Autodesk Inventor part; units mm, degrees
ref_plane "Work Plane1" through (0, 4, 5) normal (0, 0, -1) x (-1, 0, 0)
ref_plane "YZ Plane" through (0, 0, 0) normal (1, 0, 0) x (0, 1, 0)
ref_plane "XZ Plane" through (0, 0, 0) normal (0, 1, 0) x (-1, 0, 0)
sketch "Sketch1" plane through (0, 0, 0) normal (0, 1, 0) x (-1, 0, 0)
  circle A0 centre (0, 0) radius 12.7
  dimension "d0" = 25.4
extrude "Extrusion1" add sketch "Sketch1" along normal blind 4
sketch "Sketch2" plane through (0, 4, 0) normal (0, 1, 0) x (1, 0, 0)
  circle A0 centre (0, 8.382) radius 1.524
  circle A1 centre (0, 0) radius 12.7
  circle A2 centre (-8.382, 0) radius 1.524
  circle A3 centre (0, -8.382) radius 1.524
  circle A4 centre (8.382, 0) radius 1.524
  dimension "d7" = 360
extrude "Extrusion2" cut sketch "Sketch2" along normal mid plane 8 contours A0 | A2 | A3 | A4
sketch "Sketch10" plane through (0, 0, 0) normal (0, -1, 0) x (1, 0, 0)
  circle A0 centre (0, 0) radius 12.7
  circle A1 centre (0, 0) radius 3.5
  dimension "d49" = 7
extrude "Extrusion9" cut sketch "Sketch10" against normal blind 2 contours A1
sketch "Sketch11" plane through (0, 4, 0) normal (0, 1, 0) x (1, 0, 0)
  circle A0 centre (0, 0) radius 3.5
  circle A1 centre (0, 0) radius 5
  circle A2 centre (0, 0) radius 2.625
  dimension "d52" = 10
  dimension "d53" = 5.25
extrude "Extrusion10" add sketch "Sketch11" along normal blind 6 contours A0 | A1
sketch "Sketch12" plane through (0, 10, 0) normal (0, 1, 0) x (1, 0, 0)
  line L0 (0, -1.3125) -> (-2.2733, -1.3125)
  circle A0 centre (0, 0) radius 2.625
  arc A1 (-2.2733, -1.3125) -> (2.2733, -1.3125) centre (0, 0) ccw
  line L1 (0, -1.3125) -> (2.2733, -1.3125)
  dimension "d56" = 1.3125
extrude "Extrusion11" add sketch "Sketch12" against normal up to surface (6 mm away) contours L1 A0 L0 picked at (1.3942, -1.4755)
ref_plane "Work Plane1" through (0, 4, 5) normal (0, 0, -1) x (-1, 0, 0)
sketch "Sketch13" plane through (0, 4, 5) normal (0, 0, -1) x (-1, 0, 0)
  line L0 (5, 6) -> (-5, 6)
  circle A0 centre (0, 3) radius 1.25
  point P0 (0, -4)
  dimension "d60" = 2.5
extrude "Extrusion12" cut sketch "Sketch13" along normal up to surface (3.6875 mm away)
properties part number "Horn_Attachment"
Check sheet for the modelled part. Datum: model origin and axes. Units: mm. A direction names the side the tool comes from. Round coordinates to 2 decimals unless told otherwise and drop trailing zeros. Write each loop counter-clockwise with the first axis right and the second up, starting at its lowest first coordinate (ties: lowest second). Pieces come first, ordered by that corner, then holes. Notation, with made-up numbers: (-13.75, 35.5) -> (23.25, 35.5) arc R11 ccw to (23.25, 40.5) -> close; hole circle Ø7 at (38, -27). An arc over 180 degrees is marked (long way). Answer as CSV lines item,"result". Start each with the question number.
1) Material ranges on line 1 (Z direction, x = 0, y = 2.2); line 2 (Z direction, x = 0, y = 0.7); line 3 (Y direction, x = 0, z = 4.05), recorded low to high. Write a range as from..to.
2) Section check B-B on z = 0. Enter the section's corners in (x, y) (3 decimals), and give its area (3 significant figures).
3) Release check for a two-part mould opening along Z. For faces 6 (the flat face through (-5.5, 4, 0.2)), 7 (the cylindrical face through (2.75, 1.97, 12.4)), 8 (the flat face through (0, 2, 0)) record: pulls with the +Z half, pulls with the -Z half, needs draft (parallel to the pull), parting line crosses it, or undercut.
4) Section check D-D on x = -9.5. Enter the section's corners in (y, z), and give its area (3 significant figures).
5) Section check A-A on x = 0. State how many separate pieces and enclosed holes the cut face has, and give its area (3 significant figures).
6) Go/stop test with flat-tipped pins: P1, Ø6, axis at y = 7.5, z = 0.5, coming from the -X side; P2, Ø2, axis at x = -1.5, z = 1.5, coming from the -Y side; P3, Ø2, axis at x = 2.5, y = 2.5, coming from the +Z side. Record where each tip stops, or that it passes through.
7) Section check C-C on z = 7.25. Enter the section's corners in (x, y), and give its area (3 significant figures).
8) Tool access check on faces 1 (the flat face through (0, 4, 0)), 2 (the cylindrical face through (-0.33, 2.028, -6.894)), 3 (the cylindrical face through (0.27, 8.22, 3.18)), 4 (the cylindrical face through (3.233, 0.986, -1.341)), 5 (the flat face through (0, 10, 2)). Record the directions out of +Z, -Z, +X, -X, +Y, -Y that give a thin tool (end or side, any length) a straight path to the whole face; none if there is none.
Found:
1,line 1,"z = -12.7..-9.91, -6.86..6.86, 9.91..12.7"
1,line 2,"z = -12.7..-9.91, -6.86..-3.5, 3.5..6.86, 9.91..12.7"
1,line 3,"y = 0..5.75, 8.25..10"
2,outline,"(-12.7, 0) -> (-9.906, 0) -> (-9.906, 4) -> (-12.7, 4) -> close; (-6.858, 0) -> (-3.5, 0) -> (-3.5, 2) -> (3.5, 2) -> (3.5, 0) -> (6.858, 0) -> (6.858, 4) -> (5, 4) -> (5, 10) -> (2.625, 10) -> (2.625, 4) -> (-2.625, 4) -> (-2.625, 10) -> (-5, 10) -> (-5, 4) -> (-6.858, 4) -> close; (9.906, 0) -> (12.7, 0) -> (12.7, 4) -> (9.906, 4) -> close"
2,area,"91.7 mm^2"
3,face 6,"needs draft"
3,face 7,"parting line crosses it"
3,face 8,"undercut"
4,outline,"(0, -8.43) -> (4, -8.43) -> (4, -1.04) -> (0, -1.04) -> close; (0, 1.04) -> (4, 1.04) -> (4, 8.43) -> (0, 8.43) -> close"
4,area,"59.1 mm^2"
5,separate pieces,"4"
5,enclosed holes,"0"
5,area,"90.4 mm^2"
6,P1,"stops at x = -5"
6,P2,"stops at y = 2"
6,P3,"stops at z = 12.61"
7,outline,"(-10.43, 0) -> (-1.02, 0) -> (-1.02, 4) -> (-10.43, 4) -> close; (1.02, 0) -> (10.43, 0) -> (10.43, 4) -> (1.02, 4) -> close"
7,area,"75.3 mm^2"
8,face 1,"+Y"
8,face 2,"+Y, -Y"
8,face 3,"+Z"
8,face 4,"-Y"
8,face 5,"+Z, -Z, +X, -X, +Y"
